Work out the finished part from the listing and answer in its coordinate system (mm). A direction names the side the tool comes from. Coordinates: 2 decimals unless noted, no trailing zeros. Order: outer loops, then holes, each group sorted by start corner. A loop starts at its lowest first (then second) coordinate and runs counter-clockwise, first axis right, second up.
```python
from build123d import *

# Parameters (mm, degrees)
BOSS_EXTRUDE1_DEPTH = 5
SKETCH2_R           = 1.5
BOSS_EXTRUDE2_DEPTH = 6
FILLET1_R           = 0.5
SKETCH3_R           = 1.5
CUT_EXTRUDE1_DEPTH  = 2.5


with BuildPart() as part:
    # Sketch1 → Boss-Extrude1 (new body)
    with BuildSketch(Plane(origin=(0, 0, 0), x_dir=(1, 0, 0), z_dir=(0, 1, 0))):
        Polygon((3.175426481, 0), (1.58771324, 2.75), (-1.58771324, 2.75), (-3.175426481, 0), (-1.58771324, -2.75), (1.58771324, -2.75), align=None)
    extrude(amount=BOSS_EXTRUDE1_DEPTH)

    # Sketch2 → Boss-Extrude2 (add)
    with BuildSketch(Plane.XZ):
        with Locations(Location((0, 0, 0), (0, 0, 90))):
            Circle(SKETCH2_R)
    extrude(amount=BOSS_EXTRUDE2_DEPTH)

    # Fillet1
    fillet1_edges = [part.edges().sort_by_distance(p)[0] for p in [
        (0, -6, -1.5),
    ]]
    fillet(fillet1_edges, radius=FILLET1_R)

    # Sketch3 → Cut-Extrude1 (cut)
    with BuildSketch(Plane(origin=(0, 5, 0), x_dir=(1, 0, 0), z_dir=(0, 1, 0))):
        with Locations(Location((0, 0, 0), (0, 0, 270))):
            Circle(SKETCH3_R)
    extrude(amount=-CUT_EXTRUDE1_DEPTH, mode=Mode.SUBTRACT)


solid = part.part
```
1. The part is cut by section B-B (x = 0). Determine the outline of the cut face in (y, z), plus the area to 3 significant figures.
2. For faces 5 (the flat face through (1.4, 0, -1.3)), 6 (the flat face through (0, -6, 0)), determine the directions among +Z, -Z, +X, -X, +Y, -Y from which every point of the face is accessible in a straight line to the end or side of a thin tool.
3. The part is cut by section C-C (y = -3). Determine the outline of the cut face in (x, z).
4. The mould has two halves that part along X. Classify faces 1 (the cylindrical face through (0.45, 3.77, 1.43)), 2 (the flat face through (-2.37, 2.465, -1.394)), 3 (the flat face through (2.39, 2.46, -1.36)), 4 (the flat face through (0, 2.5, 0)): released by +X, released by -X, zero draft, split by the parting line, or undercut.
5. A flat-ended cylindrical pin translates along its axis: pin 1 (2.5 mm diameter, centred on x = 0, z = 0, fed in from +Y). Find the tip coordinate at first contact, or state that the pin passes through.
6. Consider probe 1 along Y at (x, z) = (1.75, -2.4); probe 2 along Z at (x, y) = (-1.25, 3); probe 3 along Z at (x, y) = (0.75, -0.5). Determine where each line is inside the solid, lowest interval first.
7. The part is cut by section D-D (y = 1.25). Determine the outline of the cut face in (x, z), plus the area to 3 significant figures.
8. The part is cut by section A-A (y = 3). Determine the outline of the cut face in (x, z).
Worked out:
1. outline: (-6, -1) arc R0.5 ccw to (-5.5, -1.5) - (0, -1.5) - (0, -2.75) - (5, -2.75) - (5, -1.5) - (2.5, -1.5) - (2.5, 1.5) - (5, 1.5) - (5, 2.75) - (0, 2.75) - (0, 1.5) - (-5.5, 1.5) arc R0.5 ccw to (-6, 1) - close
1. area: 37.9 mm2
2. face 5: -Y
2. face 6: +Z, -Z, +X, -X, -Y
3. outline: circle Ø3 at (0, 0)
4. face 1: undercut
4. face 2: released by -X
4. face 3: released by +X
4. face 4: undercut
5. pin 1: stops at y = 2.5
6. probe 1: y = 0 to 5
6. probe 2: z = -2.75 to -0.83, 0.83 to 2.75
6. probe 3: z = -1.3 to 1.3
7. outline: (-3.18, 0) - (-1.59, -2.75) - (1.59, -2.75) - (3.18, 0) - (1.59, 2.75) - (-1.59, 2.75) - close
7. area: 26.2 mm2
8. outline: (-3.18, 0) - (-1.59, -2.75) - (1.59, -2.75) - (3.18, 0) - (1.59, 2.75) - (-1.59, 2.75) - close; hole circle Ø3 at (0, 0)
